```python
from build123d import *

# Parameters (mm, degrees)
F0_W     = 190.5
F0_H     = 304.8
F1_DEPTH = 19.05
F2_R     = 38.1
F4_DEPTH = 25.4
F3_R     = 12.7
F5_DEPTH = 127


with BuildPart() as f1:
    # F0 (on Top) → F1 (new body)
    with BuildSketch(Plane.XY):
        Rectangle(F0_W, F0_H)
    extrude(amount=F1_DEPTH)

    # F2 (on face) → F4 (cut)
    with BuildSketch(Plane(origin=(0, 0, 0), x_dir=(1, 0, 0), z_dir=(0, 0, -1))):
        with Locations((0, 76.2)):
            Circle(F2_R)
    extrude(amount=-F4_DEPTH, mode=Mode.SUBTRACT)

    # F3 (on face) → F5 (join)
    with BuildSketch(Plane(origin=(0, 0, 0), x_dir=(1, 0, 0), z_dir=(0, 0, -1))):
        with Locations((0, 12.7)):
            Circle(F3_R)
    extrude(amount=F5_DEPTH)


solid = f1.part
```
Source: CAD feature listing. Evaluate the final solid. Frame: model axes, mm. Round coordinates to 2 decimals unless told otherwise and drop trailing zeros. Loops run counter-clockwise (first coordinate to the right, second up) from the corner with the lowest first, then second, coordinate; pieces in that order, holes last.
1. Section query B-B on y = -12.7. Output: boundary loops of the cut face in (x, z), and give its area (3 significant figures).
2. Mould query, pull axis X, two halves, no side actions, for faces 1 (the cylindrical face through (-1.653, -25.292, -62.611)), 2 (the flat face through (-1, 2, 19.05)), 3 (the cylindrical face through (-8.259, -39.006, 9.392)), 4 (the flat face through (95.25, -2, 9)). Classes: released by +X, released by -X, zero draft, split by the parting line, or undercut.
3. Section query A-A on x = 0. Output: boundary loops of the cut face in (y, z).
4. Contact query for a flat-ended pin moving along its axis: pin 1 (2 mm diameter, centred on x = 10, z = -58.5, fed in from -Y). Output: stop coordinate, or through.
5. Section query D-D on x = -73.5. Output: boundary loops of the cut face in (y, z), and give its area (3 significant figures).
6. Ray query, L1, parallel to Y at x = 0, z = 11.5; L2, parallel to X at y = -76.2, z = 5.25; L3, parallel to Z at x = 24, y = -3.5. Return the intervals inside material, ascending.
7. Section query C-C on z = -90. Output: boundary loops of the cut face in (x, y), and give its area (3 significant figures).
Answers below:
1. outline: (-95.25, 0) - (-12.7, 0) - (-12.7, -127) - (12.7, -127) - (12.7, 0) - (95.25, 0) - (95.25, 19.05) - (-95.25, 19.05) - close
1. area: 6,850 mm2
2. face 1: split by the parting line
2. face 2: zero draft
2. face 3: undercut
2. face 4: released by +X
3. outline: (-152.4, 0) - (-114.3, 0) - (-114.3, 19.05) - (-152.4, 19.05) - close; (-38.1, 0) - (-25.4, 0) - (-25.4, -127) - (0, -127) - (0, 0) - (152.4, 0) - (152.4, 19.05) - (-38.1, 19.05) - close
4. pin 1: stops at y = -21.66
5. outline: (-152.4, 0) - (152.4, 0) - (152.4, 19.05) - (-152.4, 19.05) - close
5. area: 5,810 mm2
6. L1: y = -152.4 to -114.3, -38.1 to 152.4
6. L2: x = -95.25 to -38.1, 38.1 to 95.25
6. L3: z = 0 to 19.05
7. outline: circle Ø25.4 at (0, -12.7)
7. area: 507 mm2
